Check sheet for the modelled part. Datum: model origin and axes. Units: mm. A direction names the side the tool comes from. Give positions to 0.01 mm unless a question says otherwise; leave off trailing zeros. Write each loop counter-clockwise with the first axis right and the second up, starting at its lowest first coordinate (ties: lowest second). Pieces come first, ordered by that corner, then holes. Notation, with made-up numbers: (12.25, -35) -> (49.25, -35) arc R35 cw to (49.25, 4) -> close; hole circle Ø5 at (-31.5, 71). An arc over 180 degrees is marked (long way). Use a Markdown table: item, result. Add a question column.
1. Set-up check for faces 1 (the flat face through (43.4, 0.11, 4.16)), 2 (the flat face through (-1, -1, 50)): record each of +Z, -Z, +X, -X, +Y, -Y from which the full face is reachable in a straight line by a thin tool's end or side.
2. Scan lines: probe 1 along Y at (x, z) = (16, 45); probe 2 along Z at (x, y) = (31, 0); probe 3 along X at (y, z) = (-5, 35). Record each from-to range of solid material in increasing order. Write a range as [from, to].
3. Cross-section at B-B (x = 34.5). Enter the section's corners in (y, z), then the cut area to 3 significant figures.
4. Release check for a two-part mould opening along Y. For faces 3 (the flat face through (-1, -1, -50)), 4 (the cylindrical face through (25.35, -0.242, 37.504)), 5 (the flat face through (-1, -50, 1)) record: released by +Y, released by -Y, zero draft, split by the parting line, or undercut.
5. Cross-section at C-C (y = 0). Enter the section's corners in (x, z).
6. Gauge pin test, flat end, axial feed: P1, Ø2, axis at y = -5.5, z = 29.5, coming from the +X side. Record the tip position at first contact, or that the pin passes through.
7. Cross-section at A-A (z = 45). Enter the section's corners in (x, y), then the cut area to 3 significant figures.
from build123d import *

# Parameters (mm, degrees)
F0_W          = 100
F0_H          = 100
F1_DEPTH      = 50
F1_DEPTH_BACK = 50
F3_R          = 7.5


with BuildPart() as f1:
    # F0 (on Front) → F1 (new body, two sides)
    with BuildSketch(Plane.XZ) as f1_sk:
        Rectangle(F0_W, F0_H)
    extrude(amount=F1_DEPTH)
    extrude(f1_sk.sketch, amount=-F1_DEPTH_BACK)

    # F4: sweep along a path in F2
    with BuildLine(Plane.XZ) as f4_path:
        Line((0, 25), (30, 25))
        Line((30, 25), (24.8696978501, 10.9046106882))
    # F3 (on Right) → F4 (sweep, cut)
    with BuildSketch(Plane.YZ):
        with Locations((0, 45)):
            Circle(F3_R)
    sweep(path=f4_path.line, transition=Transition.RIGHT, mode=Mode.SUBTRACT)


solid = f1.part
Worked answers:
| question | item | result |
|---|---|---|
| 1 | face 1 | none |
| 1 | face 2 | +Z, +X, -X, +Y, -Y |
| 2 | probe 1 | y = [-50, -7.5], [7.5, 50] |
| 2 | probe 2 | z = [-50, 37.5] |
| 2 | probe 3 | x = [-50, 48.97] |
| 3 | outline | (-50, -50) -> (50, -50) -> (50, 50) -> (5.59, 50) arc R7.5 cw (long way) to (-5.59, 50) -> (-50, 50) -> close |
| 3 | area | 9,840 mm² |
| 4 | face 3 | zero draft |
| 4 | face 4 | undercut |
| 4 | face 5 | released by -Y |
| 5 | outline | (-50, -50) -> (50, -50) -> (50, 1.76) -> (36.62, 6.63) -> (47.85, 37.5) -> (0, 37.5) -> (0, 50) -> (-50, 50) -> close |
| 6 | P1 | stops at x = 48.98 |
| 7 | outline | (-50, -50) -> (50, -50) -> (50, -7.5) -> (0, -7.5) -> (0, 7.5) -> (50, 7.5) -> (50, 50) -> (-50, 50) -> close |
| 7 | area | 9,250 mm² |
